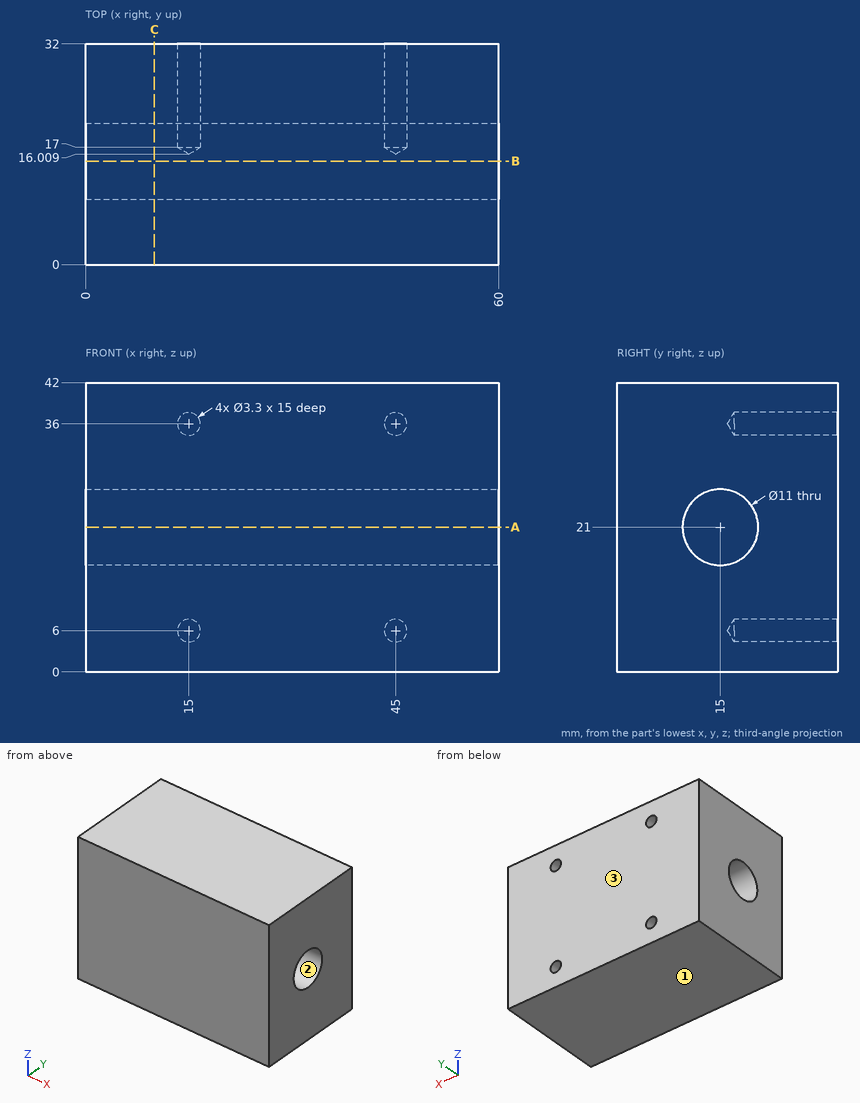
Here's the drawing with two shaded views (mm, measured from the low corner). I have some questions. Coordinates: 2 decimals unless noted, no trailing zeros. Loops run counter-clockwise (first coordinate to the right, second up) from the corner with the lowest first, then second, coordinate; pieces in that order, holes last.
Item 1: Suppose I cut it at B-B (y = 15). Please give me the cut outline in (x, z).
Answers below:
outline: (0, 0) - (60, 0) - (60, 15.5) - (0, 15.5) - close; (0, 26.5) - (60, 26.5) - (60, 42) - (0, 42) - close
Item 2: I'm going to push flat-ended pins straight in: pin 1 (3 mm diameter, centred on x = 45, z = 6, fed in from +Y); pin 2 (6.5 mm diameter, centred on y = 15, z = 21, fed in from -X) (3 decimals); pin 3 (2.5 mm diameter, centred on x = 45, z = 36, fed in from +Y). Where does each tip first touch, or does it pass through?
Answers below:
pin 1: stops at y = 16.91
pin 2: passes through
pin 3: stops at y = 16.76
Item 3: Suppose I cut it at A-A (z = 21). Please give me the cut outline in (x, y), then the cut area to 3 significant figures.
Answers below:
outline: (0, 0) - (60, 0) - (60, 9.5) - (0, 9.5) - close; (0, 20.5) - (60, 20.5) - (60, 32) - (0, 32) - close
area: 1,260 mm2
Item 4: If we mould it in two halves opening along Z, with no side actions, what happens to the marked faces 1, 2 and 3? For each: released by +Z, released by -Z, zero draft, split by the parting line, or undercut.
Answers below:
face 1: released by -Z
face 2: undercut
face 3: zero draft
Item 5: Suppose I cut it at C-C (x = 10). Please give me the cut outline in (y, z), then the cut area to 3 significant figures.
Answers below:
outline: (0, 0) - (32, 0) - (32, 42) - (0, 42) - close; hole circle Ø11 at (15, 21)
area: 1,250 mm2
Item 6: Please list where these lines run through material, in increasing order: L1, parallel to X at y = 27, z = 6; L2, parallel to Z at x = 15, y = 22.75; L3, parallel to Z at x = 16.5, y = 23 (1 decimal).
Answers below:
L1: x = 0 to 13.35, 16.65 to 43.35, 46.65 to 60
L2: z = 0 to 4.35, 7.65 to 34.35, 37.65 to 42
L3: z = 0 to 5.3, 6.7 to 35.3, 36.7 to 42
